Source: CAD feature listing. Evaluate the final solid. Frame: model axes, mm. A direction names the side the tool comes from. Round coordinates to 2 decimals unless told otherwise and drop trailing zeros. Loops run counter-clockwise (first coordinate to the right, second up) from the corner with the lowest first, then second, coordinate; pieces in that order, holes last. Notation, with made-up numbers: (84, 16) - (130, 16) arc R7 ccw to (130, 23) - close; hole circle Ø10 at (33.5, 20). An arc over 180 degrees is marked (long way). Use CSV: the item, a comma, the result in double quotes. Start each with the question number.
from build123d import *

# Parameters (mm, degrees)
BOSS_EXTRUDE1_DEPTH = 1
BOSS_EXTRUDE2_DEPTH = 6.112
CHAMFER1_SIZE       = 0.5
SKETCH3_W           = 0.5
SKETCH3_H           = 0.375
CUT_EXTRUDE1_DEPTH  = 0.3
SKETCH4_W           = 0.3
SKETCH4_H           = 1.524
BOSS_EXTRUDE3_DEPTH = 3.556
CUT_EXTRUDE2_DEPTH  = 14.276962233
FILLET1_R           = 0.3


with BuildPart() as part:
    # Sketch1 → Boss-Extrude1 (new body)
    with BuildSketch(Plane(origin=(0, 0, 0), x_dir=(0, 0, -1), z_dir=(1, 0, 0))):
        with BuildLine():
            Line((0, 0), (-2.698326862, 0))
            ThreePointArc((-2.698326862, 0), (-3.32408446, 0.336566295), (-3.388218281, 1.044193523))
            Line((-3.388218281, 1.044193523), (-1.243555187, 6.073483938))
            ThreePointArc((-1.243555187, 6.073483938), (-1.083265655, 6.857742795), (-1.243353466, 7.642042854))
            Line((-1.243353466, 7.642042854), (-2.482690665, 10.550393572))
            Line((-2.482690665, 10.550393572), (-2.206703839, 10.668))
            Line((-2.206703839, 10.668), (-0.96736664, 7.759649282))
            ThreePointArc((-0.96736664, 7.759649282), (-0.783265658, 6.857704215), (-0.967598619, 5.955806528))
            Line((-0.967598619, 5.955806528), (-3.112261714, 0.926516114))
            ThreePointArc((-3.112261714, 0.926516114), (-3.073781421, 0.501939777), (-2.698326862, 0.3))
            Line((-2.698326862, 0.3), (0, 0.3))
            Line((0, 0.3), (2.698326862, 0.3))
            ThreePointArc((2.698326862, 0.3), (3.073781421, 0.501939777), (3.112261714, 0.926516114))
            Line((3.112261714, 0.926516114), (0.967598619, 5.955806528))
            ThreePointArc((0.967598619, 5.955806528), (0.783265658, 6.857704215), (0.96736664, 7.759649282))
            Line((0.96736664, 7.759649282), (2.206703839, 10.668))
            Line((2.206703839, 10.668), (2.482690665, 10.550393572))
            Line((2.482690665, 10.550393572), (1.243353466, 7.642042854))
            ThreePointArc((1.243353466, 7.642042854), (1.083265655, 6.857742795), (1.243555187, 6.073483938))
            Line((1.243555187, 6.073483938), (3.388218281, 1.044193523))
            ThreePointArc((3.388218281, 1.044193523), (3.32408446, 0.336566295), (2.698326862, 0))
            Line((2.698326862, 0), (0, 0))
        make_face()
    extrude(amount=BOSS_EXTRUDE1_DEPTH)

    # Sketch2 → Boss-Extrude2 (add)
    with BuildSketch(Plane(origin=(1, 0, 0), x_dir=(0, 0, -1), z_dir=(1, 0, 0))):
        with BuildLine():
            Line((-1.956745691, 4.401033762), (-3.388218281, 1.044193523))
            ThreePointArc((-3.388218281, 1.044193523), (-3.32408446, 0.336566295), (-2.698326862, 0))
            Line((-2.698326862, 0), (2.698326862, 0))
            ThreePointArc((2.698326862, 0), (3.32408446, 0.336566295), (3.388218281, 1.044193523))
            Line((3.388218281, 1.044193523), (1.956745691, 4.401033762))
            ThreePointArc((1.956745691, 4.401033762), (1.945426233, 4.522631852), (2.006921941, 4.628142533))
            ThreePointArc((2.006921941, 4.628142533), (2.999999991, 6.858231733), (2.00657743, 9.088167487))
            ThreePointArc((2.00657743, 9.088167487), (1.94506764, 9.193658636), (1.956358041, 9.315249605))
            Line((1.956358041, 9.315249605), (2.482690665, 10.550393572))
            Line((2.482690665, 10.550393572), (2.206703839, 10.668))
            Line((2.206703839, 10.668), (1.680371215, 9.432856033))
            ThreePointArc((1.680371215, 9.432856033), (1.652145213, 9.128878611), (1.805919687, 8.865150738))
            ThreePointArc((1.805919687, 8.865150738), (2.699999992, 6.858208559), (1.806229747, 4.851128279))
            ThreePointArc((1.806229747, 4.851128279), (1.652490477, 4.587351579), (1.680789124, 4.283356353))
            Line((1.680789124, 4.283356353), (3.112261714, 0.926516114))
            ThreePointArc((3.112261714, 0.926516114), (3.073781421, 0.501939777), (2.698326862, 0.3))
            Line((2.698326862, 0.3), (-2.698326862, 0.3))
            ThreePointArc((-2.698326862, 0.3), (-3.073781421, 0.501939777), (-3.112261714, 0.926516114))
            Line((-3.112261714, 0.926516114), (-1.680789124, 4.283356353))
            ThreePointArc((-1.680789124, 4.283356353), (-1.652490477, 4.587351579), (-1.806229747, 4.851128279))
            ThreePointArc((-1.806229747, 4.851128279), (-2.699999992, 6.858208559), (-1.805919687, 8.865150738))
            ThreePointArc((-1.805919687, 8.865150738), (-1.652145213, 9.128878611), (-1.680371215, 9.432856033))
            Line((-1.680371215, 9.432856033), (-2.206703839, 10.668))
            Line((-2.206703839, 10.668), (-2.482690665, 10.550393572))
            Line((-2.482690665, 10.550393572), (-1.956358041, 9.315249605))
            ThreePointArc((-1.956358041, 9.315249605), (-1.94506764, 9.193658636), (-2.00657743, 9.088167487))
            ThreePointArc((-2.00657743, 9.088167487), (-2.999999991, 6.858231733), (-2.006921941, 4.628142533))
            ThreePointArc((-2.006921941, 4.628142533), (-1.945426233, 4.522631852), (-1.956745691, 4.401033762))
        make_face()
    extrude(amount=BOSS_EXTRUDE2_DEPTH)

    # Chamfer1
    chamfer1_edges = [part.edges().sort_by_distance(p)[0] for p in [
        (0, 10.609196786, 2.344697252),
        (0, 10.609196786, -2.344697252),
        (7.112, 10.609196786, -2.344697252),
        (7.112, 10.609196786, 2.344697252),
    ]]
    chamfer(chamfer1_edges, length=CHAMFER1_SIZE)

    # Sketch3 → Cut-Extrude1 (cut)
    with BuildSketch(Plane.XZ):
        with Locations((0.25, -0.9495)):
            Rectangle(SKETCH3_W, SKETCH3_H)
        with Locations((0.25, 0.9495)):
            Rectangle(SKETCH3_W, SKETCH3_H)
        with Locations((6.862, -0.9495)):
            Rectangle(SKETCH3_W, SKETCH3_H)
        with Locations((6.862, 0.9495)):
            Rectangle(SKETCH3_W, SKETCH3_H)
    extrude(amount=-CUT_EXTRUDE1_DEPTH, mode=Mode.SUBTRACT)

    # Sketch4 → Boss-Extrude3 (add)
    with BuildSketch(Plane.XZ):
        with Locations((0.15, 0)):
            Rectangle(SKETCH4_W, SKETCH4_H)
        with Locations((6.962, 0)):
            Rectangle(SKETCH4_W, SKETCH4_H)
    extrude(amount=BOSS_EXTRUDE3_DEPTH)

    # Sketch5 → Cut-Extrude2 (cut, through all)
    with BuildSketch(Plane.ZY):
        with BuildLine():
            ThreePointArc((-0.09968951, -3.556), (-0.572977926, -3.302883985), (-0.762, -2.80054914))
            Line((-0.762, -2.80054914), (-0.762, -3.556))
            Line((-0.762, -3.556), (-0.09968951, -3.556))
        make_face()
        with BuildLine():
            ThreePointArc((0.762, -2.80054914), (0.572977926, -3.302883985), (0.09968951, -3.556))
            Line((0.09968951, -3.556), (0.762, -3.556))
            Line((0.762, -3.556), (0.762, -2.80054914))
        make_face()
    extrude(amount=-CUT_EXTRUDE2_DEPTH, mode=Mode.SUBTRACT)

    # Fillet1
    fillet1_edges = [part.edges().sort_by_distance(p)[0] for p in [
        (0, 0.3, 0),
        (7.112, 0.3, 0),
    ]]
    fillet(fillet1_edges, radius=FILLET1_R)


solid = part.part
1. Contact query for flat-ended pins moving along their axis: P1, Ø4, axis at y = 6.5, z = 1, coming from the -X side; P2, Ø0.6, axis at x = 0.5, y = -0.5, coming from the -Z side; P3, Ø0.5, axis at y = 5.5, z = 1, coming from the +X side; P4, Ø0.6, axis at x = 0.5, y = -1.5, coming from the +Z side. Output: stop coordinate, or through.
2. Section query A-A on y = 0.75. Return the cut outline in (x, z), and give its area (3 significant figures).
3. Section query D-D on z = -1.5. Return the cut outline in (x, y), and give its area (3 significant figures).
4. Section query B-B on y = 7.25. Return the cut outline in (x, z), and give its area (3 significant figures).
5. Section query C-C on x = 4.5. Return the cut outline in (y, z), and give its area (3 significant figures).
6. Mould query, pull axis Y, two halves, no side actions, for faces 4 (the cylindrical face through (4, 6.9, -2.7)), 5 (the flat face through (6.812, -2, 0)), 6 (the flat face through (4, 0, 0)). Classes: +Y half, -Y half, draft (parallel to the pull), parting line (faces both ways), or undercut.
7. Line query: line 1 along Z through (x, y) = (3.75, 6.75); line 2 along Y through (x, z) = (3.75, 2.75); line 3 along Z through (x, y) = (2.25, 6). Output: solid intervals per line, ascending.
8. Reachability of faces 1 (the flat face through (0.3, -2, 0)), 2 (the cylindrical face through (0.493, 6.871, 0.783)), 3 (the cylindrical face through (0.493, 6.846, 1.083)) from +Z, -Z, +X, -X, +Y, -Y: full face, straight path, thin tool, end or side. Return the list, or none.
Values:
1,P1,"stops at x = 0"
1,P2,"stops at z = -0.76"
1,P3,"stops at x = 1"
1,P4,"stops at z = 0.76"
2,outline,"(0, -3.45) - (7.11, -3.45) - (7.11, -3.15) - (0, -3.15) - close; (0, 3.15) - (7.11, 3.15) - (7.11, 3.45) - (0, 3.45) - close"
2,area,"4.27 mm^2"
3,outline,"(0, 0) - (7.11, 0) - (7.11, 0.3) - (0, 0.3) - close; (0, 4.71) - (1, 4.71) - (1, 5.47) - (0, 5.47) - close; (0, 8.24) - (1, 8.24) - (1, 9.01) - (0, 9.01) - close"
3,area,"3.66 mm^2"
4,outline,"(0, -1.12) - (1, -1.12) - (1, -0.82) - (0, -0.82) - close; (0, 0.82) - (1, 0.82) - (1, 1.12) - (0, 1.12) - close; (1, -2.97) - (7.11, -2.97) - (7.11, -2.67) - (1, -2.67) - close; (1, 2.67) - (7.11, 2.67) - (7.11, 2.97) - (1, 2.97) - close"
4,area,"4.31 mm^2"
5,outline,"(0, -2.7) arc R0.75 ccw to (1.04, -3.39) - (4.4, -1.96) arc R0.2 cw to (4.63, -2.01) arc R3 ccw to (9.09, -2.01) arc R0.2 cw to (9.32, -1.96) - (10.55, -2.48) - (10.67, -2.21) - (9.43, -1.68) arc R0.5 ccw to (8.87, -1.81) arc R2.7 cw to (4.85, -1.81) arc R0.5 ccw to (4.28, -1.68) - (0.93, -3.11) arc R0.45 cw to (0.3, -2.7) - (0.3, 2.7) arc R0.45 cw to (0.93, 3.11) - (4.28, 1.68) arc R0.5 ccw to (4.85, 1.81) arc R2.7 cw to (8.87, 1.81) arc R0.5 ccw to (9.43, 1.68) - (10.67, 2.21) - (10.55, 2.48) - (9.32, 1.96) arc R0.2 cw to (9.09, 2.01) arc R3 ccw to (4.63, 2.01) arc R0.2 cw to (4.4, 1.96) - (1.04, 3.39) arc R0.75 ccw to (0, 2.7) - close"
5,area,"8.71 mm^2"
6,face 4,"undercut"
6,face 5,"draft"
6,face 6,"-Y half"
7,line 1,"z = -3 to -2.7, 2.7 to 3"
7,line 2,"y = 0 to 0.3, 1.78 to 2.54, 5.66 to 8.06"
7,line 3,"z = -2.87 to -2.56, 2.56 to 2.87"
8,face 1,"+Z, -Z, -Y"
8,face 2,"+X, -X"
8,face 3,"+Z, +X, -X"
